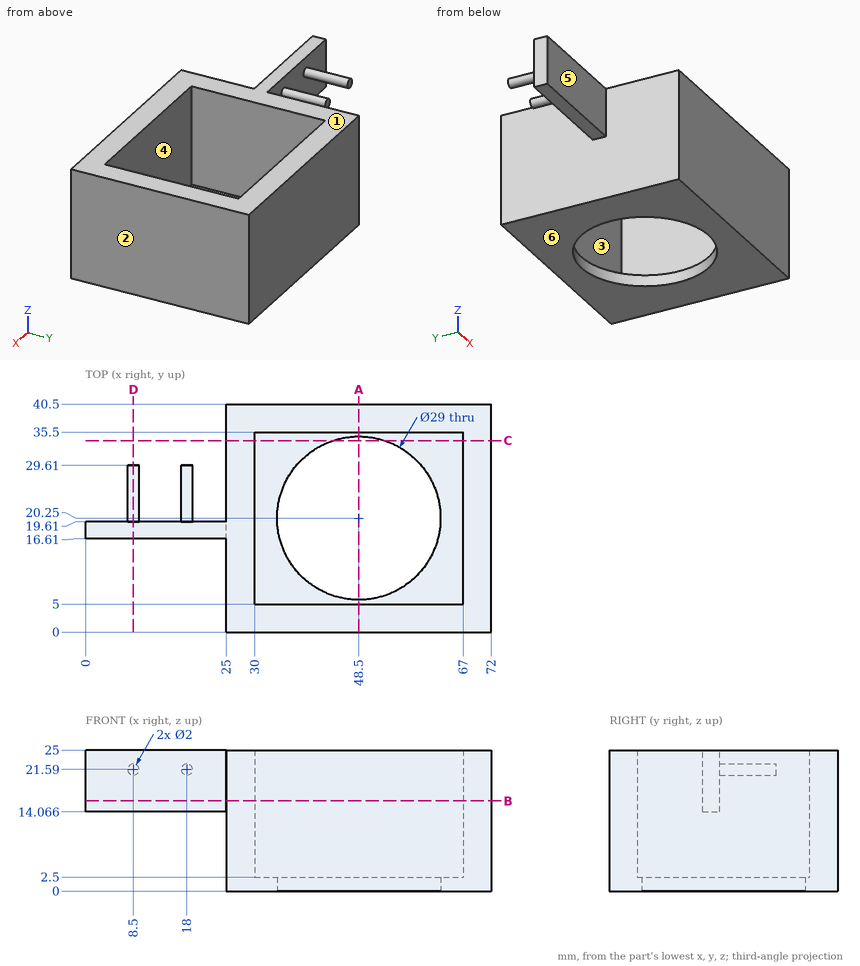
Design review of the part shown in the three views and the two pictorial views. Dimensions are in mm from the part's minimum x, y and z. A direction names the side the tool comes from. Give positions to 0.01 mm unless a question says otherwise; leave off trailing zeros. Loops run counter-clockwise (first coordinate to the right, second up) from the corner with the lowest first, then second, coordinate; pieces in that order, holes last. Notation, with made-up numbers: (-36.5, -37.5) - (-25.5, -37.5) arc R25 cw to (-25.5, -2.5) - close; hole circle Ø6 at (66.25, 62). An arc over 180 degrees is marked (long way). Write item = value, one per line.
1) Tool access review of the marked faces 4, 5 and 6: name each direction out of +Z, -Z, +X, -X, +Y, -Y from which nothing blocks a thin tool from reaching the whole face with its end or side.
Result sheet:
face_4 = +Z
face_5 = +Z, -Z, -X, -Y
face_6 = -Z, +X, -X, +Y, -Y
2) Draft analysis for pull direction X (two halves, no side actions). For the marked faces 1, 2 and 3, state which applies: +X half, -X half, draft (parallel to the pull), parting line (faces both ways), or undercut.
Result sheet:
face_1 = draft
face_2 = +X half
face_3 = undercut
3) Take a section at D-D on x = 8.5. State the section outline as (y, z) points, and give its area (3 significant figures).
Result sheet:
outline = (16.61, 14.07) - (19.61, 14.07) - (19.61, 20.59) - (29.61, 20.59) - (29.61, 22.59) - (19.61, 22.59) - (19.61, 25) - (16.61, 25) - close
area = 52.8 mm2
4) Take a section at B-B on z = 16. State the section outline as (x, y) points.
Result sheet:
outline = (0, 16.61) - (25, 16.61) - (25, 0) - (72, 0) - (72, 40.5) - (25, 40.5) - (25, 19.61) - (0, 19.61) - close; hole (30, 5) - (67, 5) - (67, 35.5) - (30, 35.5) - close
5) Take a section at A-A on x = 48.5. State the section outline as (y, z) points.
Result sheet:
outline = (0, 0) - (5.75, 0) - (5.75, 2.5) - (5, 2.5) - (5, 25) - (0, 25) - close; (34.75, 0) - (40.5, 0) - (40.5, 25) - (35.5, 25) - (35.5, 2.5) - (34.75, 2.5) - close
6) To check wall thickness, follow line 1 (Y direction, x = 42.5, z = 15.25); line 2 (X direction, y = 10, z = 22.75); line 3 (Z direction, x = 37, y = 9). State the ranges of each line that lie inside material, in increasing order.
Result sheet:
line_1 = 0 to 5, 35.5 to 40.5
line_2 = 25 to 30, 67 to 72
line_3 = 0 to 2.5
7) Take a section at C-C on y = 34. State the section outline as (x, z) points.
Result sheet:
outline = (25, 0) - (43.9, 0) - (43.9, 2.5) - (30, 2.5) - (30, 25) - (25, 25) - close; (53.1, 0) - (72, 0) - (72, 25) - (67, 25) - (67, 2.5) - (53.1, 2.5) - close
8) Clearance check with flat-ended pins moving along their axes: pin 1 Ø1.6 at (x, z) = (8, 22) entering from +Y; pin 2 Ø5.5 at (x, z) = (9, 21) entering from -Y; pin 3 Ø12 at (y, z) = (36, 12.5) entering from -X. State where each tip first meets the part, or that it passes through.
Result sheet:
pin_1 = 29.61
pin_2 = 16.61
pin_3 = 25
